from build123d import *

# Parameters (mm, degrees)
F1_DEPTH = 40
F2_W     = 101.732
F2_H     = 101.732004
F3_DEPTH = 15
F4_W     = 14
F4_H     = 20
F5_DEPTH = 10


with BuildPart() as f1:
    # F0 (on Top) → F1 (new body)
    with BuildSketch(Plane.XY):
        with BuildLine():
            Line((59.91943, 70.866002), (-71.65257, 70.866002))
            ThreePointArc((-71.65257, 70.866002), (-75.244673, 69.378105), (-76.73257, 65.786002))
            Line((-76.73257, 65.786002), (-76.73257, -65.786002))
            ThreePointArc((-76.73257, -65.786002), (-75.244673, -69.378105), (-71.65257, -70.866002))
            Line((-71.65257, -70.866002), (59.91943, -70.866002))
            ThreePointArc((59.91943, -70.866002), (63.511532, -69.378105), (64.99943, -65.786002))
            Line((64.99943, -65.786002), (64.99943, 65.786002))
            ThreePointArc((64.99943, 65.786002), (63.511532, 69.378105), (59.91943, 70.866002))
        make_face()
    extrude(amount=F1_DEPTH)

    # F2 (on face) → F3 (cut)
    with BuildSketch(Plane.XY.offset(40)):
        with Locations((-5.86657, 0)):
            Rectangle(F2_W, F2_H)
    extrude(amount=-F3_DEPTH, mode=Mode.SUBTRACT)

    # F4 (on face) → F5 (cut)
    with BuildSketch(Plane.XY.offset(40)):
        with Locations((-66.73257, 39.860209)):
            Rectangle(F4_W, F4_H)
        with Locations((-66.859915, 13.860209)):
            Rectangle(F4_W, F4_H)
        with Locations((-67.03256, -12.139791)):
            Rectangle(F4_W, F4_H)
        with Locations((54.99943, 39.860209)):
            Rectangle(F4_W, F4_H)
        with Locations((55.172075, 13.860209)):
            Rectangle(F4_W, F4_H)
        with Locations((54.99943, -12.139791)):
            Rectangle(F4_W, F4_H)
    extrude(amount=-F5_DEPTH, mode=Mode.SUBTRACT)


solid = f1.part
Verification items for the finished model (mm, model axes). A direction names the side the tool comes from. Coordinates: 2 decimals unless noted, no trailing zeros. Order: outer loops, then holes, each group sorted by start corner. A loop starts at its lowest first (then second) coordinate and runs counter-clockwise, first axis right, second up. Notation, with made-up numbers: (69, 53) -> (117, 53) arc R25 cw to (117, 92) -> close; hole circle Ø10 at (37.5, -25.75). An arc over 180 degrees is marked (long way). Use CSV: the item, a comma, the result in double quotes. Start each with the question number.
Q1. Depth check by flat-ended pin: P1, Ø1.5, axis at x = -8.5, y = -26.5, coming from the +Z side. Enter the tip coordinate at first touch or a pass-through.
Q2. Section check B-B, the plane y = -47.5. Record the cut outline in (x, z), and give its area (3 significant figures).
Q3. Section check A-A, the plane x = 2. Record the cut outline in (y, z).
Q4. Section check C-C, the plane y = 39. Record the cut outline in (x, z).
Q5. Thickness scan on line 1 along X through (y, z) = (11.5, 36); line 2 along X through (y, z) = (-10.5, 36); line 3 along Y through (x, z) = (16, 25.5). Record the ranges inside material, lowest first.
Q6. Draft check along X on faces 3 (the flat face through (-67, 23.86, 35)), 4 (the flat face through (-6, -52, 40)), 5 (the cylindrical face through (63.47, -69.42, 19.72)). Enter one of: +X half, -X half, draft (parallel to the pull), parting line (faces both ways), or undercut.
Q7. Section check D-D, the plane x = -63. Record the cut outline in (y, z).
Q8. Tool access check on faces 1 (the flat face through (55, 49.86, 35)), 2 (the flat face through (-7, 1, 0)). Record the directions out of +Z, -Z, +X, -X, +Y, -Y that give a thin tool (end or side, any length) a straight path to the whole face; none if there is none.
Returned:
1,P1,"stops at z = 25"
2,outline,"(-76.73, 0) -> (65, 0) -> (65, 40) -> (45, 40) -> (45, 25) -> (-56.73, 25) -> (-56.73, 40) -> (-76.73, 40) -> close"
2,area,"4,140 mm^2"
3,outline,"(-70.87, 0) -> (70.87, 0) -> (70.87, 40) -> (50.87, 40) -> (50.87, 25) -> (-50.87, 25) -> (-50.87, 40) -> (-70.87, 40) -> close"
4,outline,"(-76.73, 0) -> (65, 0) -> (65, 40) -> (62, 40) -> (62, 30) -> (48, 30) -> (48, 40) -> (45, 40) -> (45, 25) -> (-56.73, 25) -> (-56.73, 40) -> (-59.73, 40) -> (-59.73, 30) -> (-73.73, 30) -> (-73.73, 40) -> (-76.73, 40) -> close"
5,line 1,"x = -76.73 to -73.86, -59.86 to -56.73, 45 to 48.17, 62.17 to 65"
5,line 2,"x = -76.73 to -74.03, -60.03 to -56.73, 45 to 48, 62 to 65"
5,line 3,"y = -70.87 to -50.87, 50.87 to 70.87"
6,face 3,"undercut"
6,face 4,"draft"
6,face 5,"+X half"
7,outline,"(-70.87, 0) -> (70.87, 0) -> (70.87, 40) -> (49.86, 40) -> (49.86, 30) -> (29.86, 30) -> (29.86, 40) -> (23.86, 40) -> (23.86, 30) -> (3.86, 30) -> (3.86, 40) -> (-2.14, 40) -> (-2.14, 30) -> (-22.14, 30) -> (-22.14, 40) -> (-70.87, 40) -> close"
8,face 1,"+Z"
8,face 2,"-Z, +X, -X, +Y, -Y"
